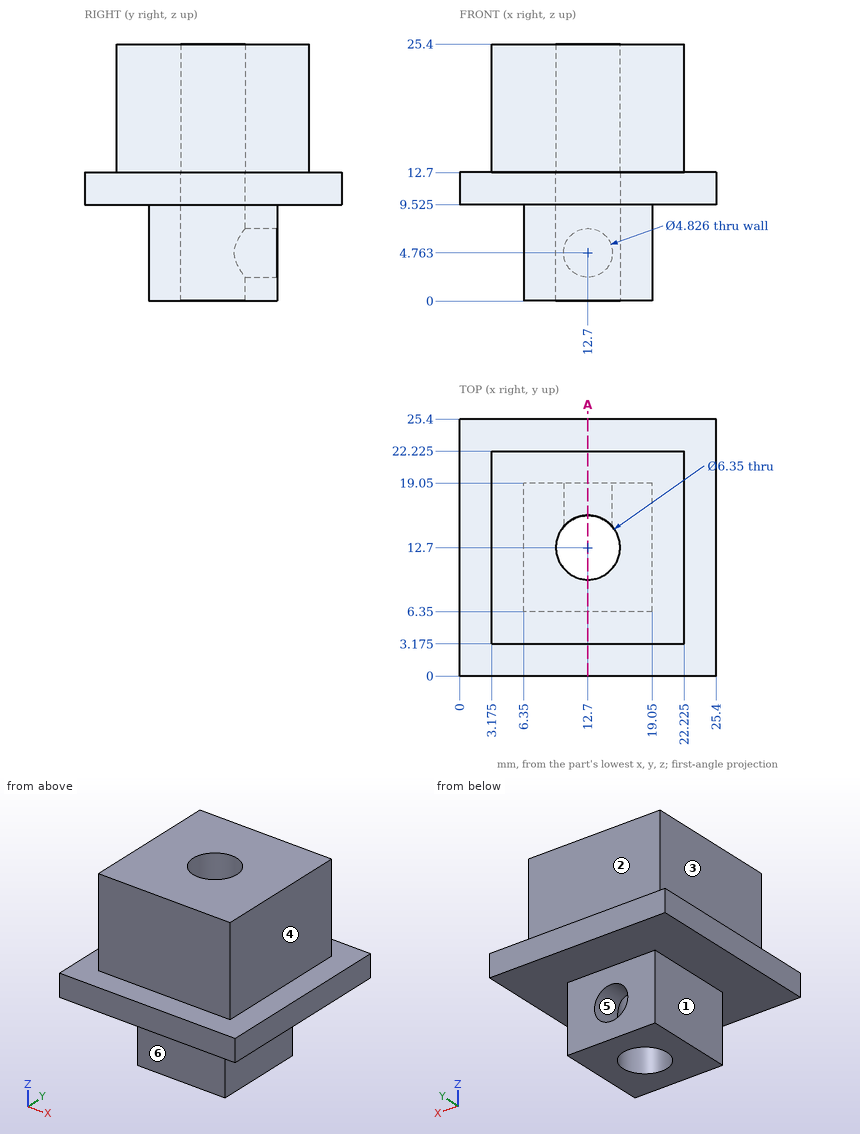
Geometry check sheet. Reference: drawing and pictorial views, mm from the part's lowest x, y, z. A direction names the side the tool comes from. Coordinates: 2 decimals unless noted, no trailing zeros.
Item 1: Access from +Z, -Z, +X, -X, +Y, -Y to the whole of each face (thin tool, end or side, straight path). Record for the marked faces 1, 2 and 3.
Filled in:
face 1: -Z, -X, +Y, -Y
face 2: +Z, +X, -X, +Y
face 3: +Z, -X, +Y, -Y
Item 2: Section check A-A, the plane x = 12.7. Give the number of separate pieces and of enclosed holes in the cut face, then the cut area to 3 significant figures.
Filled in:
separate pieces: 3
enclosed holes: 0
area: 267 mm2
Item 3: Release check for a two-part mould opening along X. For the marked faces 4, 5 and 6 record: +X half, -X half, draft (parallel to the pull), parting line (faces both ways), or undercut.
Filled in:
face 4: +X half
face 5: undercut
face 6: draft
Item 4: Material ranges on L1, parallel to Y at x = 12.7, z = 19.75 (1 decimal); L2, parallel to X at y = 4, z = 17 (1 decimal), recorded low to high.
Filled in:
L1: y = 3.2 to 9.5, 15.9 to 22.2
L2: x = 3.2 to 22.2
Item 5: Depth check by flat-ended pin: pin 1 (5 mm diameter, centred on x = 10, z = 3.5, fed in from -Y); pin 2 (4 mm diameter, centred on y = 3, z = 6.5, fed in from -X); pin 3 (1 mm diameter, centred on y = 8, z = 20.5, fed in from +X) (1 decimal); pin 4 (6.5 mm diameter, centred on x = 11, z = 20, fed in from +Y) (1 decimal). Enter the tip coordinate at first touch or a pass-through.
Filled in:
pin 1: stops at y = 6.35
pin 2: passes through
pin 3: stops at x = 22.2
pin 4: stops at y = 22.2
